For this review, take the finished solid that the model builds, in its own axes (mm). A direction names the side the tool comes from. Give positions to 0.01 mm unless a question says otherwise; leave off trailing zeros. Write each loop counter-clockwise with the first axis right and the second up, starting at its lowest first coordinate (ties: lowest second). Pieces come first, ordered by that corner, then holes. Notation, with made-up numbers: M 88.25,-25 L 95.25,-25 A16 cw 95.25,2 Z; hole C 88,21 d10. An arc over 180 degrees is marked long. One line per item, written item: value. Start each with the question number.
Item 1: Mouldability with a two-part tool opening along X and no side actions: class faces 6 (the face through (0, -32, -10)), 7 (the face through (13.5, -31, -10)), 8 (the face through (15, 33, -10)), 9 (the face through (4, 45, -3)) as released by +X, released by -X, zero draft, split by the parting line, or undercut.
Item 2: Consider section A-A, the plane y = 33. Write out the cut boundary in (x, z), and give its area (3 significant figures).
Item 3: Tool access review of faces 1 (the face through (15, -33, -10)), 2 (the face through (60, 1, 2)), 3 (the face through (8, -20, -3)), 4 (the face through (8, 31, -15)), 5 (the face through (8, 33, -20)): name each direction out of +Z, -Z, +X, -X, +Y, -Y from which nothing blocks a thin tool from reaching the whole face with its end or side.
Item 4: Consider section C-C, the plane x = 31.5. Write out the cut boundary in (y, z), and give its area (3 significant figures).
Item 5: Consider section D-D, the plane y = 15.5. Write out the cut boundary in (x, z), and give its area (3 significant figures).
Item 6: Clearance check with flat-ended pins moving along their axes: pin 1 Ø3 at (y, z) = (-32, -7.5) entering from -X; pin 2 Ø2 at (y, z) = (-34.5, -13) entering from +X; pin 3 Ø2 at (x, y) = (-7, 23.5) entering from -Z. State where each tip first meets the part, or that it passes through.
Item 7: Consider section B-B, the plane z = -9.25. Write out the cut boundary in (x, y).
Item 8: To check wall thickness, follow probe 1 along X at (y, z) = (-24.5, -10.5); probe 2 along Y at (x, z) = (14, -17); probe 3 along X at (y, z) = (-28.5, -4). State the ranges of each line that lie inside material, in increasing order.
Solid Edge part; units mm, degrees
sketch "Sketch1" plane through (0, 0, 0) normal (0, 0, 1) x (1, 0, 0)
  line L0 (0, 45) -> (60, 45)
  line L1 (60, 45) -> (60, -45)
  line L2 (60, -45) -> (-60, -45)
  line L3 (-60, -45) -> (-60, 45)
  line L4 (-60, 45) -> (0, 45)
extrude "Protrusion1" add sketch "Sketch1" along normal blind 3.5
sketch "Sketch2" plane through (0, 45, 1.75) normal (0, 1, 0) x (-1, 0, 0)
  line L0 (-15, -1.75) -> (-15, -21.75)
  line L1 (-15, -21.75) -> (0, -21.75)
  line L2 (0, -21.75) -> (0, -1.75)
  line L3 (0, -1.75) -> (-15, -1.75)
extrude "ExtrudedProtrusion_3" add sketch "Sketch2" against normal blind 25
sketch "Sketch3" plane through (7.5, 20, -10) normal (0, -1, 0) x (-1, 0, 0)
  line L0 (-6, 5) -> (6, 5)
  line L1 (6, 5) -> (6, -5)
  line L2 (6, -5) -> (-6, -5)
  line L3 (-6, -5) -> (-6, 5)
extrude "ExtrudedCutout_3" cut sketch "Sketch3" against normal blind 22
sketch "Sketch4" plane through (0, 0, 0) normal (0, 0, -1) x (-1, 0, 0)
  line L0 (0, -45) -> (-15, -45)
  line L1 (-15, -45) -> (-15, -20)
  line L2 (-15, -20) -> (0, -20)
  line L3 (0, -20) -> (0, -45)
extrude "ExtrudedProtrusion_5" add sketch "Sketch4" along normal blind 20
sketch "Sketch5" plane through (7.5, -20, -10) normal (0, 1, 0) x (-1, 0, 0)
  line L0 (-6, 5) -> (6, 5)
  line L1 (6, 5) -> (6, -5)
  line L2 (6, -5) -> (-6, -5)
  line L3 (-6, -5) -> (-6, 5)
extrude "ExtrudedCutout_4" cut sketch "Sketch5" against normal blind 22
Model answer:
1. face 6: released by -X
1. face 7: undercut
1. face 8: released by +X
1. face 9: zero draft
2. outline: M -60,0 L 0,0 L 0,-20 L 15,-20 L 15,0 L 60,0 L 60,3.5 L -60,3.5 Z; hole M 1.5,-15 L 13.5,-15 L 13.5,-5 L 1.5,-5 Z
2. area: 600 mm2
3. face 1: -Z, +X, +Y, -Y
3. face 2: +Z, -Z, +X, +Y, -Y
3. face 3: -Z, +X, -X
3. face 4: none
3. face 5: -Z, +X, -X, +Y, -Y
4. outline: M -45,0 L 45,0 L 45,3.5 L -45,3.5 Z
4. area: 315 mm2
5. outline: M -60,0 L 60,0 L 60,3.5 L -60,3.5 Z
5. area: 420 mm2
6. pin 1: stops at x = 0
6. pin 2: stops at x = 15
6. pin 3: stops at z = 0
7. outline: M 0,-45 L 15,-45 L 15,-20 L 13.5,-20 L 13.5,-42 L 1.5,-42 L 1.5,-20 L 0,-20 Z; M 0,20 L 1.5,20 L 1.5,42 L 13.5,42 L 13.5,20 L 15,20 L 15,45 L 0,45 Z
8. probe 1: x = 0 to 1.5, 13.5 to 15
8. probe 2: y = -45 to -20, 20 to 45
8. probe 3: x = 0 to 15
